Geometry check sheet. Reference: the model listing, model coordinates, mm. A direction names the side the tool comes from. Coordinates: 2 decimals unless noted, no trailing zeros. Loops run counter-clockwise (first coordinate to the right, second up) from the corner with the lowest first, then second, coordinate; pieces in that order, holes last. Notation, with made-up numbers: (-14, 43.5) -> (-7, 43.5) arc R23 cw to (-7, 65.5) -> close; hole circle Ø1 at (23.25, 23.5). An arc over 180 degrees is marked (long way). Answer as a JSON object with one key per item and string values.
from build123d import *

# Parameters (mm, degrees)
SKETCH1_R           = 2
BOSS_EXTRUDE1_DEPTH = 5
FILLET1_R           = 3


with BuildPart() as part:
    # Sketch1 → Boss-Extrude1 (new body)
    with BuildSketch(Plane(origin=(0, 0, 0), x_dir=(1, 0, 0), z_dir=(0, 1, 0))):
        with BuildLine():
            Line((-4.055, 49.113152598), (-4.055, -16.120690269))
            Line((-4.055, -16.120690269), (-4.055, -23.51992753))
            ThreePointArc((-4.055, -23.51992753), (-2.3878384, -33.44590301), (5.99940006, -27.881853402))
            Line((5.99940006, -27.881853402), (5.945, -22.441847402))
            Line((5.945, -22.441847402), (5.945, 2.058152598))
            Line((5.945, 2.058152598), (5.945, 49.113152598))
            ThreePointArc((5.945, 49.113152598), (-0.775434906, 65.337717692), (-17, 72.058152598))
            Line((-17, 72.058152598), (-17.5, 72.058152598))
            Line((-17.5, 72.058152598), (-17.5, 62.058152598))
            Line((-17.5, 62.058152598), (-17, 62.058152598))
            ThreePointArc((-17, 62.058152598), (-7.846502718, 58.26664988), (-4.055, 49.113152598))
        make_face()
        with Locations((0, -27.941847402)):
            Circle(SKETCH1_R, mode=Mode.SUBTRACT)
        with Locations((-12.5, 66.491962252)):
            Circle(SKETCH1_R, mode=Mode.SUBTRACT)
    extrude(amount=BOSS_EXTRUDE1_DEPTH)

    # Fillet1
    fillet1_edges = [part.edges().sort_by_distance(p)[0] for p in [
        (-17.5, 2.5, -62.058152598),
        (-17.5, 2.5, -72.058152598),
    ]]
    fillet(fillet1_edges, radius=FILLET1_R)


solid = part.part
1. Section check C-C, the plane z = -28.5. Record the boundary of the cut face in (x, y) (3 decimals), then the cut area to 3 significant figures.
Evaluation:
{"outline": "(-4.055, 0) -> (5.945, 0) -> (5.945, 5) -> (-4.055, 5) -> close", "area": "50.0 mm^2"}
2. Thickness scan on probe 1 along X at (y, z) = (4.1, 27.5); probe 2 along X at (y, z) = (3.9, 19) (3 decimals); probe 3 along Z at (x, y) = (0, 2.5). Record the ranges inside material, lowest first. Write a range as from..to.
Evaluation:
{"probe 1": "x = -5.98..-1.95, 1.95..6", "probe 2": "x = -4.055..5.945", "probe 3": "z = -64.52..25.94, 29.94..33.94"}
3. Section check D-D, the plane x = -12.5. Record the boundary of the cut face in (y, z).
Evaluation:
{"outline": "(0, -71.61) -> (5, -71.61) -> (5, -68.49) -> (0, -68.49) -> close; (0, -64.49) -> (5, -64.49) -> (5, -61.25) -> (0, -61.25) -> close"}
4. Section check B-B, the plane y = 2.25. State how many separate pieces and enclosed holes the cut face has, then the cut area to 3 significant figures.
Evaluation:
{"separate pieces": "1", "enclosed holes": "2", "area": "1,090 mm^2"}
5. Depth check by flat-ended pin: P1, Ø1.5, axis at x = 1.5, y = 3.5, coming from the -Z side; P2, Ø12, axis at x = -7, z = -31.5, coming from the +Y side; P3, Ø1.5, axis at y = 2.5, z = -9.5, coming from the +X side (3 decimals). Enter the tip coordinate at first touch or a pass-through.
Evaluation:
{"P1": "stops at z = -63.65", "P2": "stops at y = 5", "P3": "stops at x = 5.945"}
6. Mould release check, pull along Z, two halves, no side actions. Record for faces 1 (the face through (0.364, 2.465, -64.112)), 2 (the face through (-7.24, 2.46, -57.62)), 3 (the face through (-1, 5, -20)): released by +Z, released by -Z, zero draft, split by the parting line, or undercut.
Evaluation:
{"face 1": "released by -Z", "face 2": "undercut", "face 3": "zero draft"}
7. Tool access check on faces 4 (the face through (-1, 0, -20)), 5 (the face through (-4.055, 2, -13)). Record the directions out of +Z, -Z, +X, -X, +Y, -Y that give a thin tool (end or side, any length) a straight path to the whole face; none if there is none.
Evaluation:
{"face 4": "+Z, -Z, +X, -X, -Y", "face 5": "-X, +Y, -Y"}
8. Section check A-A, the plane x = 0.75. Record the boundary of the cut face in (y, z), then the cut area to 3 significant figures.
Evaluation:
{"outline": "(0, -63.65) -> (5, -63.65) -> (5, 26.09) -> (0, 26.09) -> close; (0, 29.8) -> (5, 29.8) -> (5, 33.89) -> (0, 33.89) -> close", "area": "469 mm^2"}
